Source: three-view drawing plus pictorial views. Frame: mm from the lowest corner of the part. A direction names the side the tool comes from. Round coordinates to 2 decimals unless told otherwise and drop trailing zeros. Loops run counter-clockwise (first coordinate to the right, second up) from the corner with the lowest first, then second, coordinate; pieces in that order, holes last. Notation, with made-up numbers: (56, 36.25) -> (107, 36.25) arc R24 cw to (107, 58.25) -> close; hole circle Ø4 at (10.5, 24.5). An arc over 180 degrees is marked (long way). Answer in a Markdown table with one row per item.
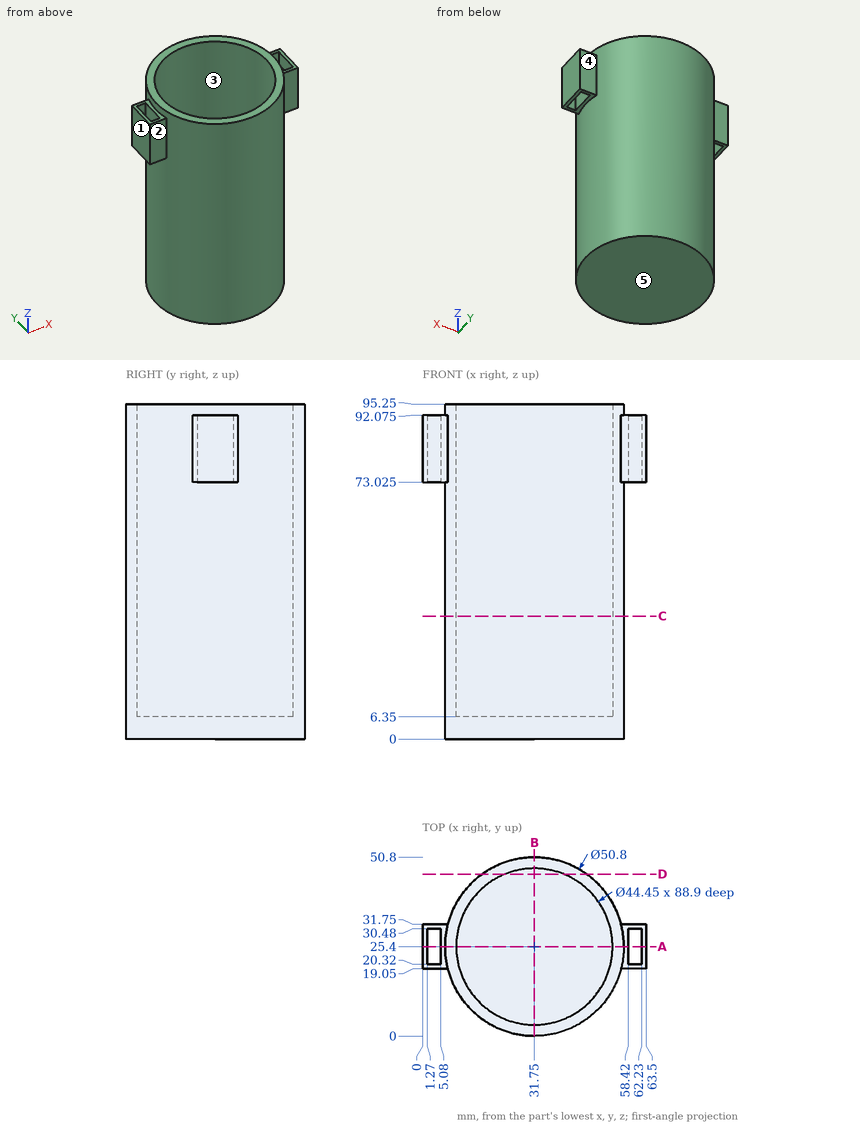
Item 1: Pin query (flat end, axial travel): pin 1 Ø4 at (x, z) = (57, 66) entering from -Y; pin 2 Ø6 at (y, z) = (44.5, 19.5) entering from +X; pin 3 Ø2 at (x, z) = (3.5, 80.5) entering from -Y. Return the tip coordinate at first contact, or that it passes through.
Answer:
| item | result |
|---|---|
| pin 1 | stops at y = 15.17 |
| pin 2 | stops at x = 51.4 |
| pin 3 | stops at y = 19.05 |
Item 2: Cut plane A-A (y = 25.4). Output: boundary loops of the cut face in (x, z) (3 decimals), then the cut area to 3 significant figures.
Answer:
| item | result |
|---|---|
| outline | (0, 73.025) -> (1.27, 73.025) -> (1.27, 92.075) -> (0, 92.075) -> close; (5.08, 73.025) -> (6.35, 73.025) -> (6.35, 0) -> (57.15, 0) -> (57.15, 73.025) -> (58.42, 73.025) -> (58.42, 92.075) -> (57.15, 92.075) -> (57.15, 95.25) -> (53.975, 95.25) -> (53.975, 6.35) -> (9.525, 6.35) -> (9.525, 95.25) -> (6.35, 95.25) -> (6.35, 92.075) -> (5.08, 92.075) -> close; (62.23, 73.025) -> (63.5, 73.025) -> (63.5, 92.075) -> (62.23, 92.075) -> close |
| area | 984 mm² |
Item 3: Cut plane C-C (z = 35). Output: boundary loops of the cut face in (x, y) (3 decimals), then the cut area to 3 significant figures.
Answer:
| item | result |
|---|---|
| outline | circle Ø50.8 at (31.75, 25.4); hole circle Ø44.45 at (31.75, 25.4) |
| area | 475 mm² |
Item 4: Reachability of the marked faces 4 and 5 from +Z, -Z, +X, -X, +Y, -Y: full face, straight path, thin tool, end or side. Return the list, or none.
Answer:
| item | result |
|---|---|
| face 4 | +Z, -Z, +X, +Y |
| face 5 | -Z, +X, -X, +Y, -Y |
Item 5: Line query: probe 1 along X at (y, z) = (25, 46); probe 2 along Z at (x, y) = (18, 10); probe 3 along Y at (x, z) = (17.5, 60). Output: solid intervals per line, ascending. Write a range as [from, to].
Answer:
| item | result |
|---|---|
| probe 1 | x = [6.35, 9.53], [53.97, 57.15] |
| probe 2 | z = [0, 6.35] |
| probe 3 | y = [4.37, 8.34], [42.46, 46.43] |
Item 6: Cut plane B-B (x = 31.75). Output: boundary loops of the cut face in (y, z) (3 decimals), then the cut area to 3 significant figures.
Answer:
| item | result |
|---|---|
| outline | (0, 0) -> (50.8, 0) -> (50.8, 95.25) -> (47.625, 95.25) -> (47.625, 6.35) -> (3.175, 6.35) -> (3.175, 95.25) -> (0, 95.25) -> close |
| area | 887 mm² |
Item 7: Draft query along Y for the marked faces 1, 2 and 3. Return one class per face: pulls with the +Y half, pulls with the -Y half, needs draft (parallel to the pull), parting line crosses it, or undercut.
Answer:
| item | result |
|---|---|
| face 1 | needs draft |
| face 2 | pulls with the -Y half |
| face 3 | undercut |
Item 8: Cut plane D-D (y = 46). Output: boundary loops of the cut face in (x, z), then the cut area to 3 significant figures.
Answer:
| item | result |
|---|---|
| outline | (16.89, 0) -> (46.61, 0) -> (46.61, 95.25) -> (40.09, 95.25) -> (40.09, 6.35) -> (23.41, 6.35) -> (23.41, 95.25) -> (16.89, 95.25) -> close |
| area | 1,350 mm² |
